Check sheet for the modelled part. Datum: model origin and axes. Units: mm. A direction names the side the tool comes from. Round coordinates to 2 decimals unless told otherwise and drop trailing zeros. Loops run counter-clockwise (first coordinate to the right, second up) from the corner with the lowest first, then second, coordinate; pieces in that order, holes last. Notation, with made-up numbers: (89, 18.25) - (141, 18.25) arc R4 cw to (141, 23.25) - close; hole circle Ø10 at (3, 11.5). An arc over 180 degrees is marked (long way). Put each result on its own line as item: value. Start each with the question number.
```python
from build123d import *

# Parameters (mm, degrees)
SKETCH_W        = 145
SKETCH_H        = 60
PAD_DEPTH       = 30
THICKNESS_T     = -2
SKETCH001_W     = 141
SKETCH001_H     = 56
PAD001_DEPTH    = 1.5
SKETCH002_W     = 30
SKETCH002_H     = 25
POCKET_DEPTH    = 2
SKETCH003_W     = 5
SKETCH003_H     = 30
POCKET001_DEPTH = 3.5
SKETCH004_R     = 1.5
PAD002_DEPTH    = 4


with BuildPart() as part:
    # Sketch → Pad (new body)
    with BuildSketch(Plane.XY):
        Rectangle(SKETCH_W, SKETCH_H)
    extrude(amount=PAD_DEPTH)

    # Thickness
    thickness_openings = [part.faces().sort_by_distance(p)[0] for p in [
        (0, 0, 30),
    ]]
    offset(amount=THICKNESS_T, openings=thickness_openings, kind=Kind.INTERSECTION)

    # Sketch001 (on Face5 of Thickness) → Pad001 (join)
    with BuildSketch(Plane(origin=(0, 0, 0), x_dir=(1, 0, 0), z_dir=(0, 0, -1))):
        Rectangle(SKETCH001_W, SKETCH001_H)
    extrude(amount=PAD001_DEPTH)

    # Sketch002 (on Face2 of Pad001) → Pocket (cut)
    with BuildSketch(Plane(origin=(-72.5, 0, 0), x_dir=(0, -1, 0), z_dir=(-1, 0, 0))):
        with Locations((0, 17.5)):
            Rectangle(SKETCH002_W, SKETCH002_H)
    extrude(amount=-POCKET_DEPTH, mode=Mode.SUBTRACT)

    # Sketch003 (on Face19 of Pocket) → Pocket001 (cut)
    with BuildSketch(Plane.XY.offset(2)):
        with Locations((57.5, 0)):
            Rectangle(SKETCH003_W, SKETCH003_H)
    extrude(amount=-POCKET001_DEPTH, mode=Mode.SUBTRACT)

    # Sketch004 (on Face19 of Pocket001) → Pad002 (join)
    with BuildSketch(Plane.XY.offset(2)):
        with Locations((-35.5, 24.15)):
            Circle(SKETCH004_R)
        with Locations((-36.8, -24.15)):
            Circle(SKETCH004_R)
        with Locations((39.4, 24.15)):
            Circle(SKETCH004_R)
        with Locations((15.3, -19.05)):
            Circle(SKETCH004_R)
    extrude(amount=PAD002_DEPTH)


solid = part.part
```
Q1. Cross-section at A-A on y = -2. Enter the section's corners in (x, z).
Q2. Depth check by flat-ended pin: pin 1 Ø2.5 at (x, y) = (15, -19) entering from +Z; pin 2 Ø12 at (x, y) = (-36, -7) entering from +Z; pin 3 Ø0.6 at (x, y) = (-71.5, 3) entering from +Z. Enter the tip coordinate at first touch or a pass-through.
Q3. Set-up check for faces 4 (the face through (-1, 0, -1.5)), 5 (the face through (-70.5, 0, 3)), 6 (the face through (57, 15, 0)): record each of +Z, -Z, +X, -X, +Y, -Y from which the full face is reachable in a straight line by a thin tool's end or side.
Q4. Cross-section at D-D on z = 26. Enter the section's corners in (x, y), and give its area (3 significant figures).
Q5. Cross-section at B-B on y = 18.5. Enter the section's corners in (x, z).
Q6. Cross-section at C-C on x = 15.3. Enter the section's corners in (y, z), and give its area (3 significant figures).
Q7. Draft check along Y on faces 1 (the face through (-72.5, -0.4, 4.8)), 2 (the face through (16.73, -18.6, 3.97)), 3 (the face through (55, 0, 0)). Enter one of: +Y half, -Y half, draft (parallel to the pull), parting line (faces both ways), or undercut.
Q8. Material ranges on line 1 (Y direction, x = 46.5, z = 9.5); line 2 (X direction, y = -16.5, z = 27); line 3 (Z direction, x = 13.5, y = 10), recorded low to high. Write a range as from..to.
Answer list:
1. outline: (-72.5, 0) - (-70.5, 0) - (-70.5, -1.5) - (55, -1.5) - (55, 2) - (-70.5, 2) - (-70.5, 5) - (-72.5, 5) - close; (60, -1.5) - (70.5, -1.5) - (70.5, 0) - (72.5, 0) - (72.5, 30) - (70.5, 30) - (70.5, 2) - (60, 2) - close
2. pin 1: stops at z = 6
2. pin 2: stops at z = 2
2. pin 3: stops at z = 5
3. face 4: -Z, +X, -X, +Y, -Y
3. face 5: +Z
3. face 6: +Z, -Z
4. outline: (-72.5, -30) - (72.5, -30) - (72.5, 30) - (-72.5, 30) - (-72.5, 15) - (-70.5, 15) - (-70.5, 28) - (70.5, 28) - (70.5, -28) - (-70.5, -28) - (-70.5, -15) - (-72.5, -15) - close
4. area: 744 mm2
5. outline: (-72.5, 0) - (-70.5, 0) - (-70.5, -1.5) - (70.5, -1.5) - (70.5, 0) - (72.5, 0) - (72.5, 30) - (70.5, 30) - (70.5, 2) - (-70.5, 2) - (-70.5, 30) - (-72.5, 30) - close
6. outline: (-30, 0) - (-28, 0) - (-28, -1.5) - (28, -1.5) - (28, 0) - (30, 0) - (30, 30) - (28, 30) - (28, 2) - (-17.55, 2) - (-17.55, 6) - (-20.55, 6) - (-20.55, 2) - (-28, 2) - (-28, 30) - (-30, 30) - close
6. area: 328 mm2
7. face 1: draft
7. face 2: undercut
7. face 3: undercut
8. line 1: y = -30..-28, 28..30
8. line 2: x = -72.5..-70.5, 70.5..72.5
8. line 3: z = -1.5..2
